from build123d import *

# Parameters (mm, degrees)
CROQUIS1_R              = 5
CROQUIS1_R_2            = 3.275
SALIENTE_EXTRUIR1_DEPTH = 3.25
CROQUIS3_R              = 5
CROQUIS3_R_2            = 2.25
SALIENTE_EXTRUIR2_DEPTH = 2
REDONDEO1_R             = 0.6
REDONDEO2_R             = 1
CHAFL_N1_SIZE           = 0.7
CHAFL_N2_SIZE           = 0.5
SKETCH1_W               = 13.933828458
SKETCH1_H               = 2
CUT_EXTRUDE1_DEPTH      = 2
SKETCH2_R               = 3.25
CUT_EXTRUDE2_DEPTH      = 1.5
SKETCH3_W               = 17.261868402
SKETCH3_H               = 2
CUT_EXTRUDE3_DEPTH      = 3
CUT_EXTRUDE4_REACH      = 11.437
SKETCH4_W               = 4.736283822
SKETCH4_H               = 4.25
FILLET1_R               = 1


with BuildPart() as part:
    # Croquis1 → Saliente-Extruir1 (new body)
    with BuildSketch(Plane(origin=(0, 0, 0), x_dir=(1, 0, 0), z_dir=(0, 1, 0))):
        with Locations(Location((0, 0, 0), (0, 0, 90))):
            Circle(CROQUIS1_R)
        with Locations(Location((0, 0, 0), (0, 0, 90))):
            Circle(CROQUIS1_R_2, mode=Mode.SUBTRACT)
    extrude(amount=SALIENTE_EXTRUIR1_DEPTH)

    # Croquis2 → Revolución1 (revolve)
    with BuildSketch(Plane.XY, mode=Mode.PRIVATE) as revoluci_n1_sk:
        Polygon((-5, 3.25), (-5, 4.25), (-2.25, 4.25), (-2.25, 4.15), (-3.275, 3.25), align=None)
    revolve(revoluci_n1_sk.sketch.rotate(Axis((0, 0, 0), (0, 1, 0)), 270), axis=Axis((0, 0, 0), (0, 1, 0)))

    # Croquis3 → Saliente-Extruir2 (add)
    with BuildSketch(Plane(origin=(0, 4.25, 0), x_dir=(1, 0, 0), z_dir=(0, 1, 0))):
        with Locations(Location((0, 0, 0), (0, 0, 90))):
            Circle(CROQUIS3_R)
        with Locations(Location((0, 0, 0), (0, 0, 90))):
            Circle(CROQUIS3_R_2, mode=Mode.SUBTRACT)
    extrude(amount=SALIENTE_EXTRUIR2_DEPTH)

    # Redondeo1
    redondeo1_edges = [part.edges().sort_by_distance(p)[0] for p in [
        (0, 6.25, 5),
    ]]
    fillet(redondeo1_edges, radius=REDONDEO1_R)

    # Redondeo2
    redondeo2_edges = [part.edges().sort_by_distance(p)[0] for p in [
        (0, 4.15, 2.25),
    ]]
    fillet(redondeo2_edges, radius=REDONDEO2_R)

    # Chaflán1
    chafl_n1_edges = [part.edges().sort_by_distance(p)[0] for p in [
        (0, 0, 3.275),
    ]]
    chamfer(chafl_n1_edges, length=CHAFL_N1_SIZE)

    # Chaflán2
    chafl_n2_edges = [part.edges().sort_by_distance(p)[0] for p in [
        (0, 6.25, 2.25),
    ]]
    chamfer(chafl_n2_edges, length=CHAFL_N2_SIZE)

    # Sketch1 → Cut-Extrude1 (cut)
    with BuildSketch(Plane(origin=(0, 6.25, 0), x_dir=(1, 0, 0), z_dir=(0, 1, 0))):
        Rectangle(SKETCH1_W, SKETCH1_H)
    extrude(amount=-CUT_EXTRUDE1_DEPTH, mode=Mode.SUBTRACT)

    # Sketch2 → Cut-Extrude2 (cut)
    with BuildSketch(Plane(origin=(0, 6.25, 0), x_dir=(1, 0, 0), z_dir=(0, 1, 0))):
        Circle(SKETCH2_R)
    extrude(amount=-CUT_EXTRUDE2_DEPTH, mode=Mode.SUBTRACT)

    # Sketch3 → Cut-Extrude3 (cut)
    with BuildSketch(Plane.XZ):
        Rectangle(SKETCH3_W, SKETCH3_H)
    extrude(amount=-CUT_EXTRUDE3_DEPTH, mode=Mode.SUBTRACT)

    # Cut-Extrude4: up to this face of the body (flat: up to its plane)
    cut_extrude4_end = Plane(part.part.faces().sort_by_distance((3.602612573, 4.25, -9.08e-07))[0])
    # Sketch4 → Cut-Extrude4 (cut, up to the picked face)
    with BuildSketch(Plane(origin=(0, 6.25, 0), x_dir=(1, 0, 0), z_dir=(0, 1, 0)), mode=Mode.PRIVATE) as cut_extrude4_sk1:
        with Locations((-3.541734363, 0)):
            Rectangle(SKETCH4_W, SKETCH4_H)
    cut_extrude4_tool1 = split(extrude(cut_extrude4_sk1.sketch, amount=-CUT_EXTRUDE4_REACH, mode=Mode.PRIVATE), bisect_by=cut_extrude4_end, keep=Keep.BOTH, mode=Mode.PRIVATE)
    add(cut_extrude4_tool1.solids().sort_by(Axis((-3.541734, 6.25, 0), (0, -1, 0)))[0], mode=Mode.SUBTRACT)

    # Fillet1
    fillet1_edges = [part.edges().sort_by_distance(p)[0] for p in [
        (4.008786459, 3, -1),
        (-4.008786459, 3, -1),
        (4.008786459, 3, 1),
        (-4.008786459, 3, 1),
    ]]
    fillet(fillet1_edges, radius=FILLET1_R - 0.0001)  # a hair under: the kernel refuses the full size


solid = part.part
For this review, take the finished solid that the model builds, in its own axes (mm). A direction names the side the tool comes from. Coordinates: 2 decimals unless noted, no trailing zeros. Write each loop counter-clockwise with the first axis right and the second up, starting at its lowest first coordinate (ties: lowest second). Pieces come first, ordered by that corner, then holes. Notation, with made-up numbers: (-12, 88.5) -> (9, 88.5) arc R8 ccw to (9, 93.5) -> close; hole circle Ø1 at (35.25, 76.5). An arc over 180 degrees is marked (long way). Write each question's results on one line, items separated by ' | '. Start each with the question number.
1) Insertion check: pin 1 (1 mm diameter, centred on x = -3, y = 5.5, fed in from -Z); pin 2 (1 mm diameter, centred on x = 3, y = 5.5, fed in from +Z); pin 3 (2 mm diameter, centred on x = 4, y = 1, fed in from -Z). Each pin has a flat end and moves straight along its axis. Give the tip position at first contact, or say it passes through.
2) Consider section A-A (y = 1.5). Write out the cut boundary in (x, z) (3 decimals), plus the area to 3 significant figures.
3) For faces 4 (the face through (-3, 5, -2.125)), 5 (the face through (-4, 1, 1)), 6 (the face through (0.2, 6.25, -3.4)), 7 (the face through (0.063, 0.578, -3.396)), 8 (the face through (0.598, 5.51, 3.194)), list the 3-axis set-ups (+Z, -Z, +X, -X, +Y, -Y) from which the entire face can be reached by the end or side of a thin tool; tool diameter is ignored.
4) The part is to be moulded in two halves that separate along X. For faces 1 (the face through (4.88, 2.79, 1.08)), 2 (the face through (0.3, 4.75, -2.4)), 3 (the face through (4.072, 2.715, -0.699)), say which applies: +X half, -X half, draft (parallel to the pull), parting line (faces both ways), or undercut.
5) Wall thickness on L1, parallel to X at y = 2.75, z = 3; L2, parallel to Z at x = 1.5, y = 2.25; L3, parallel to Z at x = -2.5, y = 4.75 (3 decimals): over which ranges is each line inside the solid? List them lowest first. Write a range as [from, to].
Geometry says:
1) pin 1: z = -4.33 | pin 2: z = 4.33 | pin 3: z = -4
2) outline: (-4.899, -1) arc R5 ccw to (4.899, -1) -> (3.119, -1) arc R3.275 cw to (-3.119, -1) -> close; (-4.899, 1) -> (-3.119, 1) arc R3.275 cw to (3.119, 1) -> (4.899, 1) arc R5 ccw to start | area: 37.9 mm^2
3) face 4: -X, +Y | face 5: +X, -X, -Y | face 6: +Z, -Z, +X, -X, +Y | face 7: -Y | face 8: +Y
4) face 1: parting line | face 2: undercut | face 3: draft
5) L1: [-4, -1.31], [1.31, 4] | L2: [-4.77, -2.91], [2.91, 4.77] | L3: [-4.33, -2.125], [2.125, 4.33]
